The listing builds one solid part. Answer for the finished solid, in the listing's coordinates (mm). Round coordinates to 2 decimals unless told otherwise and drop trailing zeros. Order: outer loops, then holes, each group sorted by start corner. A loop starts at its lowest first (then second) coordinate and runs counter-clockwise, first axis right, second up. Notation, with made-up numbers: M 31.5,-7.75 L 64.5,-7.75 A27 cw 64.5,13.25 Z; hole C -21.75,-9.75 d7. An arc over 180 degrees is marked long. Write item = value, one per line. Start each with the question number.
(1) A cutting plane is placed at A-A, the plane y = 125. Determine the outline of the cut face in (x, z).
(2) Straight lines are drawn through the part: probe 1 along Z at (x, y) = (0, 1.5); probe 2 along Z at (x, y) = (12.5, 77); probe 3 along Y at (x, z) = (49.5, 49). For each, find the intervals that lie inside material, in ascending order. Write a range as from..to.
(3) Each of these flat-tipped pins is pushed along its axis until it touches: pin 1 (18 mm diameter, centred on x = -49, z = -54, fed in from -Y); pin 2 (12 mm diameter, centred on x = -47, z = -33.5, fed in from -Y); pin 3 (1 mm diameter, centred on x = -53.5, y = 87.5, fed in from +Z); pin 4 (6 mm diameter, centred on x = -52, y = 39, fed in from +Z). Where does it stop, or does it pass through?
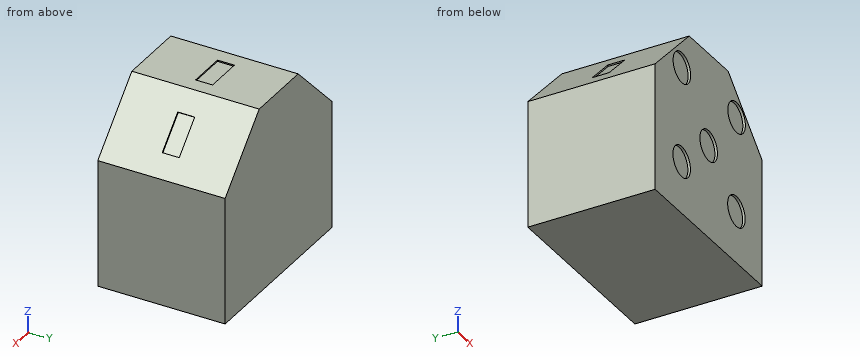
Autodesk Inventor part; units mm, degrees
ref_plane "YZ Plane" through (0, 0, 0) normal (1, 0, 0) x (0, 1, 0)
ref_plane "XZ Plane" through (0, 0, 0) normal (0, 1, 0) x (-1, 0, 0)
ref_plane "XY Plane" through (0, 0, 0) normal (0, 0, 1) x (1, 0, 0)
sketch "Sketch1" plane through (0, 0, 0) normal (0, 1, 0) x (-1, 0, 0)
  line L0 (110, -110) -> (-110, -110)
  line L1 (-110, -110) -> (-110, 110)
  line L2 (-110, 110) -> (110, 110)
  line L3 (110, 110) -> (110, -110)
  dimension "d2" = 220
  dimension "d3" = 220
extrude "Extrusion1" add sketch "Sketch1" along normal blind 150
sketch "Sketch2" plane through (-110, 0, 110) normal (0, 0, 1) x (1, 0, 0)
  line L0 (220, 150) -> (0, 150)
  line L1 (0, 0) -> (220, 0)
  line L2 (0, 0) -> (0, 150)
  line L3 (87.5, 85) -> (132.5, 85)
  line L4 (132.5, 85) -> (132.5, 65)
  line L5 (132.5, 65) -> (87.5, 65)
  line L6 (87.5, 65) -> (87.5, 85)
  line L7 (87.5, 85) -> (132.5, 65) construction
  line L8 (132.5, 85) -> (87.5, 65) construction
  point P0 (110, 0)
  point P1 (110, 75)
  dimension "d6" = 45
  dimension "d7" = 20
extrude "Extrusion2" cut sketch "Sketch2" against normal blind 1.5
chamfer "Chamfer1" distance 70 angle 45 2 edges at (110, 75, 110) (-110, 75, 110)
sketch "Sketch3" plane through (40, 0, 110) normal (0.7071, 0, 0.7071) x (0.7071, 0, -0.7071)
  line L0 (26.9975, 65) -> (71.9975, 65)
  line L1 (71.9975, 65) -> (71.9975, 85)
  line L2 (71.9975, 85) -> (26.9975, 85)
  line L3 (26.9975, 85) -> (26.9975, 65)
  line L4 (26.9975, 65) -> (71.9975, 85) construction
  line L5 (71.9975, 65) -> (26.9975, 85) construction
  point P0 (49.4975, 75)
  dimension "d13" = 45
  dimension "d14" = 20
extrude "Extrusion3" cut sketch "Sketch3" against normal blind 1.5
sketch "Sketch4" plane through (-110, 0, 40) normal (-0.7071, 0, 0.7071) x (0.7071, 0, 0.7071)
  line L0 (26.9975, 85) -> (71.9975, 85)
  line L1 (71.9975, 85) -> (71.9975, 65)
  line L2 (71.9975, 65) -> (26.9975, 65)
  line L3 (26.9975, 65) -> (26.9975, 85)
  line L4 (26.9975, 85) -> (71.9975, 65) construction
  line L5 (71.9975, 85) -> (26.9975, 65) construction
  point P0 (49.4975, 75)
  dimension "d17" = 45
  dimension "d18" = 20
extrude "Extrusion4" cut sketch "Sketch4" against normal blind 1.5
sketch "Sketch5" plane through (0, 0, 0) normal (0, -1, 0) x (1, 0, 0)
  circle A0 centre (-55.0452, 64.279) radius 18
  circle A1 centre (0, 0) radius 18
  circle A2 centre (0, 0) radius 18
  circle A3 centre (57.3798, 63.8751) radius 18
  circle A4 centre (-55.4491, -48.146) radius 18
  circle A5 centre (56.9759, -48.5499) radius 18
extrude "Extrusion7" cut sketch "Sketch5" against normal blind 3
properties part number "bodyy"
Reported:
q1.outline = M -110,-110 L 110,-110 L 110,40 L 40,110 L -40,110 L -110,40 Z
q2.probe_1 = -110..-18, 18..110
q2.probe_2 = -110..108.5
q2.probe_3 = 3..150
q3.pin_1 = 3
q3.pin_2 = 0
q3.pin_3 = 97
q3.pin_4 = 101
